Geometry check sheet. Reference: the model listing, model coordinates, mm. A direction names the side the tool comes from. Round coordinates to 2 decimals unless told otherwise and drop trailing zeros. Order: outer loops, then holes, each group sorted by start corner. A loop starts at its lowest first (then second) coordinate and runs counter-clockwise, first axis right, second up. Notation, with made-up numbers: (-31, 4.5) - (2, 4.5) arc R6 ccw to (2, 14.5) - close; hole circle Ø9 at (57.25, 54.5). An arc over 180 degrees is marked (long way). One line per question, with ' | ' between items. Start each with the question number.
Q1. Sectioned sample at D-D, the plane x = 12.25. Enter the section's corners in (y, z).
Q2. Tool access check on faces 1 (the face through (13.609, 5.135, 1.14)), 2 (the face through (5.598, 23.535, 0.088)), 3 (the face through (5.2, -1.2, -23.5)), 4 (the face through (3.6, 14.9, -14.8)), 5 (the face through (4, 0, 21)). Record the directions out of +Z, -Z, +X, -X, +Y, -Y that give a thin tool (end or side, any length) a straight path to the whole face; none if there is none.
Q3. Gauge pin test, flat ends, axial feed: P1, Ø5, axis at x = 4.5, y = -10, coming from the -Z side; P2, Ø12, axis at x = 3.5, y = -13, coming from the -Z side; P3, Ø2, axis at x = 3, z = 0.5, coming from the -Y side. Record the tip position at first contact, or that the pin passes through.
Q4. Material ranges on line 1 along X through (y, z) = (10, 21.5); line 2 along Y through (x, z) = (12.75, 2); line 3 along Y through (x, z) = (11.25, 1), recorded low to high.
Q5. Sectioned sample at A-A, the plane z = 0. Enter the section's corners in (x, y), then the cut area to 3 significant figures.
Q6. Mould release check, pull along Y, two halves, no side actions. Record for faces 6 (the face through (4, 21, 0)), 7 (the face through (5.598, -23.535, -0.088)), 8 (the face through (4.03, 18.02, 15.26)), 9 (the face through (12.347, 3.212, 0.713)): +Y half, -Y half, draft (parallel to the pull), parting line (faces both ways), or undercut.
```python
from build123d import *

# Parameters (mm, degrees)
SKETCH2_R          = 2
CUT_EXTRUDE1_DEPTH = 5
CIRPATTERN1_COUNT  = 8


with BuildPart() as part:
    # Sketch1 → Revolve2 (revolve)
    with BuildSketch(Plane.XY, mode=Mode.PRIVATE) as revolve2_sk:
        Polygon((7.2, 26), (0, 26), (0, 18), (6.2, 2), (7.2, 2), (20.2, 5.26), (7.2, 5.26), align=None)
    revolve(revolve2_sk.sketch.rotate(Axis((20.2, 0, 0), (-1, 0, 0)), 90), axis=Axis((20.2, 0, 0), (-1, 0, 0)))

    # Sketch2 → Cut-Extrude1 (cut)
    with BuildSketch(Plane(origin=(0, 0, -26), x_dir=(-1, 0, 0), z_dir=(0, 0, -1))):
        with Locations((-3.6, 0)):
            Circle(SKETCH2_R)
    cut_extrude1 = extrude(amount=-CUT_EXTRUDE1_DEPTH, mode=Mode.SUBTRACT)

    # CirPattern1: Cut-Extrude1 ×8 about axis
    cirpattern1_axis = Axis((0, 0, 0), (1, 0, 0))
    for i in range(1, CIRPATTERN1_COUNT):
        add(cut_extrude1.rotate(cirpattern1_axis, i * 360 / CIRPATTERN1_COUNT), mode=Mode.SUBTRACT)


solid = part.part
```
Determined:
1) outline: circle Ø10.52 at (0, 0); hole circle Ø6.53 at (0, 0)
2) face 1: +X | face 2: +Y | face 3: -Z | face 4: none | face 5: +Z
3) P1: stops at z = -24.89 | P2: stops at z = -25.04 | P3: stops at y = -21
4) line 1: x = 0 to 7.2 | line 2: y = -4.86 to -2.74, 2.74 to 4.86 | line 3: y = -5.16 to -2.84, 2.84 to 5.16
5) outline: (0, -26) - (1.6, -26) - (1.6, -21) - (5.6, -21) - (5.6, -26) - (7.2, -26) - (7.2, -5.26) - (20.2, -5.26) - (7.2, -2) - (6.2, -2) - (0, -18) - close; (0, 18) - (6.2, 2) - (7.2, 2) - (20.2, 5.26) - (7.2, 5.26) - (7.2, 26) - (5.6, 26) - (5.6, 21) - (1.6, 21) - (1.6, 26) - (0, 26) - close | area: 249 mm2
6) face 6: +Y half | face 7: draft | face 8: undercut | face 9: undercut
